Geometry check sheet. Reference: drawing and pictorial views, mm from the part's lowest x, y, z. A direction names the side the tool comes from. Give positions to 0.01 mm unless a question says otherwise; leave off trailing zeros. Loops run counter-clockwise (first coordinate to the right, second up) from the corner with the lowest first, then second, coordinate; pieces in that order, holes last. Notation, with made-up numbers: (31, -8.5) - (69, -8.5) arc R21 ccw to (69, 14.5) - close; hole circle Ø8 at (-38.5, 22.25). An arc over 180 degrees is marked (long way). Answer in a Markdown table with one row per item. Add a question column.
(1) Sectioned sample at B-B on y = 30. Enter the section's corners in (x, z), then the cut area to 3 significant figures.
(2) Sectioned sample at A-A on x = 2.5. Enter the section's corners in (y, z), then the cut area to 3 significant figures.
(3) Set-up check for the marked faces 1, 2 and 3: record each of +Z, -Z, +X, -X, +Y, -Y from which the full face is reachable in a straight line by a thin tool's end or side.
(4) Thickness scan on L1, parallel to Z at x = 2.5, y = 30; L2, parallel to Y at x = 16.5, z = 4.25; L3, parallel to X at y = 29.3, z = 5. Record the ranges inside material, lowest first.
(5) Go/stop test with flat-tipped pins: P1, Ø6, axis at x = 2.5, z = 15, coming from the -Y side; P2, Ø5, axis at x = 41.5, z = 4.5, coming from the +Y side; P3, Ø3, axis at y = 35, z = 7, coming from the -X side; P4, Ø4, axis at y = 8, z = 6, coming from the +X side. Record where each tip stops, or that it passes through.
(6) Sectioned sample at D-D on x = 36. Enter the section's corners in (y, z), then the cut area to 3 significant figures.
(7) Sectioned sample at C-C on z = 3.25. Enter the section's corners in (x, y), then the cut area to 3 significant figures.
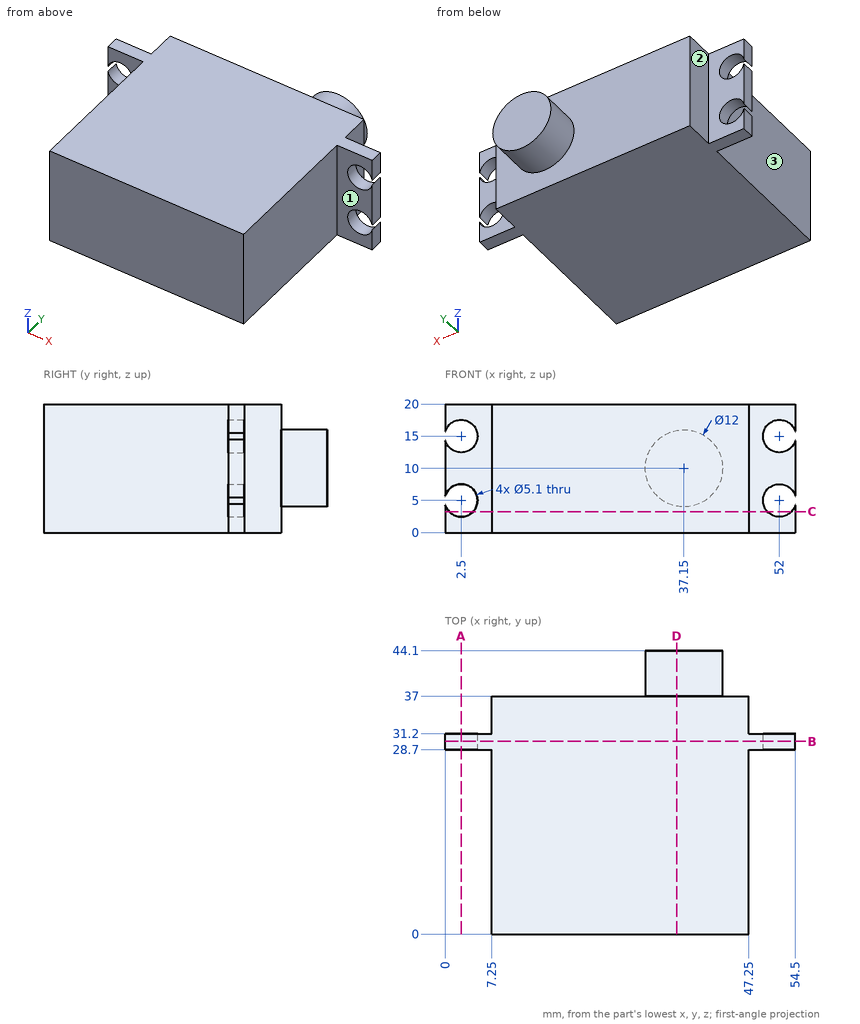
Reply:
| question | item | result |
|---|---|---|
| 1 | outline | (0, 0) - (54.5, 0) - (54.5, 4.5) arc R2.55 cw (long way) to (54.5, 5.5) - (54.5, 14.5) arc R2.55 cw (long way) to (54.5, 15.5) - (54.5, 20) - (0, 20) - (0, 15.5) arc R2.55 cw (long way) to (0, 14.5) - (0, 5.5) arc R2.55 cw (long way) to (0, 4.5) - close |
| 1 | area | 1,010 mm^2 |
| 2 | outline | (28.7, 0) - (31.2, 0) - (31.2, 2.45) - (28.7, 2.45) - close; (28.7, 7.55) - (31.2, 7.55) - (31.2, 12.45) - (28.7, 12.45) - close; (28.7, 17.55) - (31.2, 17.55) - (31.2, 20) - (28.7, 20) - close |
| 2 | area | 24.5 mm^2 |
| 3 | face 1 | +Z, -Z, +X, -Y |
| 3 | face 2 | +Z, -Z, -X, +Y |
| 3 | face 3 | +Z, -Z, -X, -Y |
| 4 | L1 | 0 to 2.45, 7.55 to 12.45, 17.55 to 20 |
| 4 | L2 | 0 to 37 |
| 4 | L3 | 5.05 to 49.45 |
| 5 | P1 | y = 28.7 |
| 5 | P2 | y = 44.1 |
| 5 | P3 | x = 7.25 |
| 5 | P4 | x = 47.25 |
| 6 | outline | (0, 0) - (37, 0) - (37, 4.11) - (44.1, 4.11) - (44.1, 15.89) - (37, 15.89) - (37, 20) - (0, 20) - close |
| 6 | area | 824 mm^2 |
| 7 | outline | (0, 28.7) - (0.65, 28.7) - (0.65, 31.2) - (0, 31.2) - close; (4.35, 28.7) - (7.25, 28.7) - (7.25, 0) - (47.25, 0) - (47.25, 28.7) - (50.15, 28.7) - (50.15, 31.2) - (47.25, 31.2) - (47.25, 37) - (7.25, 37) - (7.25, 31.2) - (4.35, 31.2) - close; (53.85, 28.7) - (54.5, 28.7) - (54.5, 31.2) - (53.85, 31.2) - close |
| 7 | area | 1,500 mm^2 |
